```python
from build123d import *

# Parameters (mm, degrees)
F1_DEPTH = 16.764
F3_DEPTH = 6.35
F4_W     = 43.18
F4_H     = 3.81
F5_DEPTH = 3.81
F7_DEPTH = 1.27


with BuildPart() as f1:
    # F0 (on Front) → F1 (new body)
    with BuildSketch(Plane.XZ):
        Polygon((-25.4, -6.35), (0, -6.35), (25.4, -6.35), (25.4, 0), (-25.4, 0), align=None)
    extrude(amount=F1_DEPTH)

    # F2 (on face) → F3 (join)
    with BuildSketch(Plane.XY):
        Polygon((-25.4, 0), (-25.4, -16.764), (-21.59, -16.764), (-21.59, -3.81), (0, -3.81), (21.59, -3.81), (21.59, -16.764), (25.4, -16.764), (25.4, 0), align=None)
    extrude(amount=F3_DEPTH)

    # F4 (on face) → F5 (join)
    with BuildSketch(Plane.XY.offset(6.35)):
        with Locations((0, -1.905)):
            Rectangle(F4_W, F4_H)
    extrude(amount=F5_DEPTH)

    # F6 (on face) → F7 (join)
    with BuildSketch(Plane.XY.offset(6.35)):
        Polygon((-25.4, -12.954), (-25.4, -16.764), (-25.4, -20.574), (-12.7, -20.574), (-12.7, -12.954), align=None)
    extrude(amount=F7_DEPTH)

    # F8: F1 across plane


with BuildPart() as f1_1:
    add(f1.part)
    add(f1.part.mirror(Plane.YZ))


solid = f1_1.part
```
CAD build for the part. Positions are in the model's coordinates, mm. A direction names the side the tool comes from. Round coordinates to 2 decimals unless told otherwise and drop trailing zeros. Order: outer loops, then holes, each group sorted by start corner. A loop starts at its lowest first (then second) coordinate and runs counter-clockwise, first axis right, second up. Notation, with made-up numbers: (19.5, 17) - (28.5, 17) arc R18 ccw to (28.5, 41) - close; hole circle Ø1 at (85.5, 25.5). An arc over 180 degrees is marked (long way). Answer as CSV lines item,"result". Start each with the question number.
1. Saw through at C-C, the plane y = -18.5. Write the cut outline in (x, z), and give its area (3 significant figures).
2. Saw through at A-A, the plane x = 15.5. Write the cut outline in (y, z), and give its area (3 significant figures).
3. Pin check, flat tips, straight feed: pin 1 (3 mm diameter, centred on x = 24, y = -5.5, fed in from +Z); pin 2 (8.5 mm diameter, centred on x = -19, y = -16.5, fed in from +Z); pin 3 (4 mm diameter, centred on x = -6.5, y = -9, fed in from +Z). Stop position of each tip, or through.
4. Saw through at D-D, the plane y = -15.5. Write the cut outline in (x, z), and give its area (3 significant figures).
5. Drill centre lines: L1, parallel to X at y = -7.5, z = 2.5; L2, parallel to Z at x = -17, y = -14.25; L3, parallel to Y at x = -16, z = 7. Where is each one in solid material? Low to high. Write a range as [from, to].
6. Pull direction Y, two halves, no side cores. Call faces 5 (the face through (-18, -17, 6.35)), 6 (the face through (-19, -12.954, 7)), 7 (the face through (-19, -20.574, 7)): +Y half, -Y half, draft (parallel to the pull), parting line (faces both ways), or undercut.
7. Saw through at B-B, the plane z = 3.5. Write the cut outline in (x, y).
8. Tool access for faces 1 (the face through (23, -6, 6.35)), 2 (the face through (12.7, -17, 7)), 3 (the face through (21.59, -10, 3)), 4 (the face through (19, -17, 7.62)): list every direction of +Z, -Z, +X, -X, +Y, -Y with a clear straight run to the whole face (end or side of a thin tool).
Model answer:
1,outline,"(-25.4, 6.35) - (-12.7, 6.35) - (-12.7, 7.62) - (-25.4, 7.62) - close; (12.7, 6.35) - (25.4, 6.35) - (25.4, 7.62) - (12.7, 7.62) - close"
1,area,"32.3 mm²"
2,outline,"(-20.57, 6.35) - (-12.95, 6.35) - (-12.95, 7.62) - (-20.57, 7.62) - close; (-16.76, -6.35) - (0, -6.35) - (0, 10.16) - (-3.81, 10.16) - (-3.81, 0) - (-16.76, 0) - close"
2,area,"155 mm²"
3,pin 1,"stops at z = 6.35"
3,pin 2,"stops at z = 7.62"
3,pin 3,"stops at z = 0"
4,outline,"(-25.4, -6.35) - (25.4, -6.35) - (25.4, 7.62) - (12.7, 7.62) - (12.7, 6.35) - (21.59, 6.35) - (21.59, 0) - (-21.59, 0) - (-21.59, 6.35) - (-12.7, 6.35) - (-12.7, 7.62) - (-25.4, 7.62) - close"
4,area,"403 mm²"
5,L1,"x = [-25.4, -21.59], [21.59, 25.4]"
5,L2,"z = [-6.35, 0], [6.35, 7.62]"
5,L3,"y = [-20.57, -12.95], [-3.81, 0]"
6,face 5,"draft"
6,face 6,"undercut"
6,face 7,"-Y half"
7,outline,"(-25.4, -16.76) - (-21.59, -16.76) - (-21.59, -3.81) - (21.59, -3.81) - (21.59, -16.76) - (25.4, -16.76) - (25.4, 0) - (-25.4, 0) - close"
8,face 1,"+Z, +X, +Y"
8,face 2,"+Z, -Y"
8,face 3,"-Y"
8,face 4,"+Z, +X, -X, -Y"
